CAD build for the part. Positions are in the model's coordinates, mm. A direction names the side the tool comes from. Coordinates: 2 decimals unless noted, no trailing zeros. Order: outer loops, then holes, each group sorted by start corner. A loop starts at its lowest first (then second) coordinate and runs counter-clockwise, first axis right, second up. Notation, with made-up numbers: (2, 32.5) - (39, 32.5) arc R11 cw to (39, 51.5) - close; hole circle Ø5 at (9, 51.25). An arc over 180 degrees is marked (long way). Use one line per item in the form item = value.
```python
from build123d import *

# Parameters (mm, degrees)
SKETCH2_W           = 114.3
SKETCH2_H           = 50.8
SKETCH2_W_2         = 88.9
SKETCH2_H_2         = 25.4
BOSS_EXTRUDE1_DEPTH = 12.7
FILLET3_R           = 25.4
FILLET4_R           = 12.7
SKETCH5_W           = 31.75
SKETCH5_H           = 12.7
BOSS_EXTRUDE2_DEPTH = 28.575
FILLET5_R           = 15.875
SKETCH6_R           = 6.35
CUT_EXTRUDE1_DEPTH  = 124.825
SKETCH7_W           = 31.75
SKETCH7_H           = 12.7
CUT_EXTRUDE2_DEPTH  = 129.30300318


with BuildPart() as part:
    # Sketch2 → Boss-Extrude1 (new body)
    with BuildSketch(Plane(origin=(0, 0, 0), x_dir=(1, 0, 0), z_dir=(0, 1, 0))):
        with Locations((57.15, 25.4)):
            Rectangle(SKETCH2_W, SKETCH2_H)
        with Locations((57.15, 25.4)):
            Rectangle(SKETCH2_W_2, SKETCH2_H_2, mode=Mode.SUBTRACT)
    extrude(amount=-BOSS_EXTRUDE1_DEPTH)

    # Fillet3
    fillet3_edges = [part.edges().sort_by_distance(p)[0] for p in [
        (0, -6.35, 0),
        (0, -6.35, -50.8),
        (114.3, -6.35, -50.8),
        (114.3, -6.35, 0),
    ]]
    fillet(fillet3_edges, radius=FILLET3_R - 0.0001)  # a hair under: the kernel refuses the full size

    # Fillet4
    fillet4_edges = [part.edges().sort_by_distance(p)[0] for p in [
        (12.7, -6.35, -12.7),
        (101.6, -6.35, -12.7),
        (101.6, -6.35, -38.1),
        (12.7, -6.35, -38.1),
    ]]
    fillet(fillet4_edges, radius=FILLET4_R - 0.0001)  # a hair under: the kernel refuses the full size

    # Sketch5 → Boss-Extrude2 (add)
    with BuildSketch(Plane(origin=(0, 0, 0), x_dir=(1, 0, 0), z_dir=(0, 1, 0))):
        with Locations((57.15, 44.45)):
            Rectangle(SKETCH5_W, SKETCH5_H)
    extrude(amount=BOSS_EXTRUDE2_DEPTH)

    # Fillet5
    fillet5_edges = [part.edges().sort_by_distance(p)[0] for p in [
        (41.275, 28.575, -44.45),
        (73.025, 28.575, -44.45),
    ]]
    fillet(fillet5_edges, radius=FILLET5_R - 0.0001)  # a hair under: the kernel refuses the full size

    # Sketch6 → Cut-Extrude1 (cut, through all)
    with BuildSketch(Plane.XY.offset(-38.1)):
        with Locations((57.15, 12.7)):
            Circle(SKETCH6_R)
    extrude(amount=-CUT_EXTRUDE1_DEPTH, mode=Mode.SUBTRACT)

    # Sketch7 → Cut-Extrude2 (cut, through all)
    with BuildSketch(Plane(origin=(0, 0, 0), x_dir=(1, 0, 0), z_dir=(0, 1, 0))):
        with Locations((57.15, 6.35)):
            Rectangle(SKETCH7_W, SKETCH7_H)
    extrude(amount=-CUT_EXTRUDE2_DEPTH, mode=Mode.SUBTRACT)


solid = part.part
```
Item 1: Drill centre lines: line 1 (Y direction, x = 57.15, z = -46) (3 decimals); line 2 (Z direction, x = 80.5, y = -5); line 3 (Z direction, x = 46, y = -5). Where is each one in solid material? Low to high. Write a range as [from, to].
Derived:
line_1 = [-12.7, 6.35], [19.05, 28.575]
line_2 = [-50.8, -38.1], [-12.7, 0]
line_3 = [-50.8, -38.1]
Item 2: Cut at B-B, the plane z = -6. Write the cut outline in (x, y) (3 decimals), plus the area to 3 significant figures.
Derived:
outline = (9.005, -12.7) - (41.275, -12.7) - (41.275, 0) - (9.005, 0) - close; (73.025, -12.7) - (105.295, -12.7) - (105.295, 0) - (73.025, 0) - close
area = 820 mm²
Item 3: Cut at D-D, the plane x = 45. Write the cut outline in (y, z), plus the area to 3 significant figures.
Derived:
outline = (-12.7, -50.8) - (22.92, -50.8) - (22.92, -38.1) - (-12.7, -38.1) - close
area = 452 mm²
Item 4: 3-axis set-ups, long thin cutter, end or side, ignore diameter. For faces 1 (the face through (73.025, 6, -44)), 2 (the face through (81, -6, -12.7)), 3 (the face through (41.275, -6, -6)): which of +Z, -Z, +X, -X, +Y, -Y reach the whole face in a straight line?
Derived:
face_1 = +Z, -Z, +X, +Y
face_2 = +Y, -Y
face_3 = +Z, +Y, -Y
Item 5: Two-plate mould, pull along X, no slides. Class faces 4 (the face through (41.275, 6, -44)), 5 (the face through (97.98, -6.44, -34.28)), 6 (the face through (103, 0, -26)), 7 (the face through (106.66, -6.44, -7.24)): +X half, -X half, draft (parallel to the pull), parting line (faces both ways), or undercut.
Derived:
face_4 = -X half
face_5 = undercut
face_6 = draft
face_7 = +X half
Item 6: Cut at A-A, the plane x = 30. Write the cut outline in (y, z).
Derived:
outline = (-12.7, -50.8) - (0, -50.8) - (0, -38.1) - (-12.7, -38.1) - close; (-12.7, -12.7) - (0, -12.7) - (0, 0) - (-12.7, 0) - close
Item 7: Drop flat-ended pins along their axis: pin 1 (6.5 mm diameter, centred on y = -4.5, z = -6, fed in from +X); pin 2 (8 mm diameter, centred on y = 1, z = -30, fed in from +X); pin 3 (1.5 mm diameter, centred on y = -1, z = -19, fed in from +X). Give the stop position or say it passes through.
Derived:
pin_1 = 108.5
pin_2 = 114.29
pin_3 = 113.66
